Can you work these out from the model? Positions are in its coordinate system, mm. Face numbers are marked on the shaded views. A direction names the side the tool comes from. Coordinates: 2 decimals unless noted, no trailing zeros. Order: outer loops, then holes, each group sorted by start corner. A loop starts at its lowest first (then second) coordinate and runs counter-clockwise, first axis right, second up. Notation, with made-up numbers: (22.25, 16) -> (73.25, 16) arc R13 cw to (73.25, 41) -> close; hole circle Ø1 at (0, 69.25). An arc over 180 degrees is marked (long way). Use a Markdown table: item, result. Add a question column.
1. Suppose I cut it at B-B, the plane z = -12. List the corners of the cut face in (x, y) for me.
2. We'd pull the mould along Z, two halves only. Please class the marked faces 3, 4 and 5: pulls with the +Z half, pulls with the -Z half, needs draft (parallel to the pull), parting line crosses it, or undercut.
3. If I drill on line 1 along Y through (x, z) = (-28.5, -2); line 2 along Y through (x, z) = (35, -16); line 3 along Z through (x, y) = (-12.5, 304), over which ranges is the centre line in solid material (lowest first)? Write a range as from..to.
4. Suppose I cut it at C-C, the plane x = 0. List the corners of the cut face in (y, z) for me.
5. For the marked faces 1 and 2, which set-ups out of +Z, -Z, +X, -X, +Y, -Y let a thin tool reach every point of the face, with its end or its side?
6. For pin 1 Ø2 at (y, z) = (340, 31.5) entering from +X; pin 2 Ø12 at (y, z) = (303.5, -22) entering from +X; pin 3 Ø5.5 at (y, z) = (42.5, 26.5) entering from -X; pin 4 Ø5 at (x, z) = (-13.5, 31.5) entering from -Y, each with a flat end and sliding along its axis, tell me the tip position at first contact or that it passes through.
7. Suppose I cut it at D-D, the plane y = 258. List the corners of the cut face in (x, z) for me.
8. Suppose I cut it at A-A, the plane y = 320.5. List the corners of the cut face in (x, z) for me.
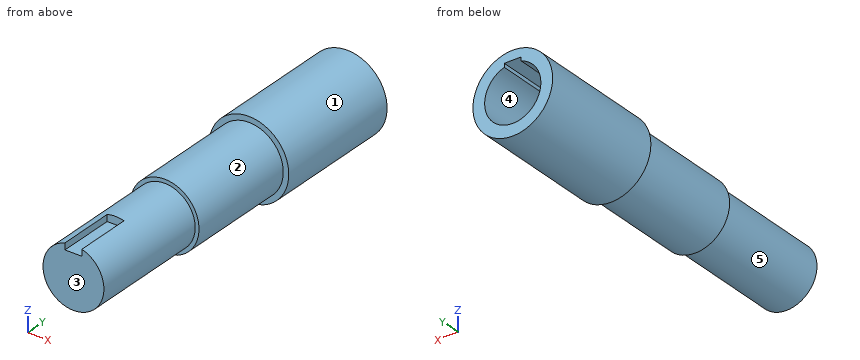
```python
from build123d import *

# Parameters (mm, degrees)
F0_R      = 32.5
F1_DEPTH  = 100
F2_R      = 36.5851523514
F3_DEPTH  = 150
F4_R      = 42.5
F5_DEPTH  = 140
F7_DEPTH  = 110
F9_DEPTH  = 60
F10_R     = 36.5851523514
F10_R_2   = 32.5
F11_DEPTH = 30


with BuildPart() as f1:
    # F0 (on Front) → F1 (new body)
    with BuildSketch(Plane.XZ):
        Circle(F0_R)
    extrude(amount=-F1_DEPTH)

    # F2 (on face) → F3 (join)
    with BuildSketch(Plane(origin=(0, 100, 0), x_dir=(-1, 0, 0), z_dir=(0, 1, 0))):
        Circle(F2_R)
    extrude(amount=F3_DEPTH)

    # F4 (on face) → F5 (join)
    with BuildSketch(Plane(origin=(0, 250, 0), x_dir=(-1, 0, 0), z_dir=(0, 1, 0))):
        Circle(F4_R)
    extrude(amount=F5_DEPTH)

    # F6 (on face) → F7 (cut)
    with BuildSketch(Plane(origin=(0, 390, 0), x_dir=(-1, 0, 0), z_dir=(0, 1, 0))):
        with BuildLine():
            Line((-9, 32.6181760425), (-9, 28.6181760425))
            ThreePointArc((-9, 28.6181760425), (0, -30), (9, 28.6181760425))
            Line((9, 28.6181760425), (9, 32.6181760425))
            Line((9, 32.6181760425), (-9, 32.6181760425))
        make_face()
    extrude(amount=-F7_DEPTH, mode=Mode.SUBTRACT)

    # F8 (on face) → F9 (cut)
    with BuildSketch(Plane.XZ):
        with BuildLine():
            ThreePointArc((9, 31.2289929393), (0, 32.5), (-9, 31.2289929393))
            Line((-9, 31.2289929393), (-9, 24.2289929393))
            Line((-9, 24.2289929393), (9, 24.2289929393))
            Line((9, 24.2289929393), (9, 31.2289929393))
        make_face()
    extrude(amount=-F9_DEPTH, mode=Mode.SUBTRACT)

    # F10 (on face) → F11 (cut)
    with BuildSketch(Plane.XZ.offset(-100)):
        Circle(F10_R)
        Circle(F10_R_2, mode=Mode.SUBTRACT)
    extrude(amount=-F11_DEPTH, mode=Mode.SUBTRACT)


solid = f1.part
```
Worked out:
| question | item | result |
|---|---|---|
| 1 | outline | (-40.77, 250) -> (-34.56, 250) -> (-34.56, 130) -> (-30.2, 130) -> (-30.2, 0) -> (30.2, 0) -> (30.2, 130) -> (34.56, 130) -> (34.56, 250) -> (40.77, 250) -> (40.77, 390) -> (27.5, 390) -> (27.5, 280) -> (-27.5, 280) -> (-27.5, 390) -> (-40.77, 390) -> close |
| 2 | face 3 | needs draft |
| 2 | face 4 | undercut |
| 2 | face 5 | parting line crosses it |
| 3 | line 1 | y = 0..280 |
| 3 | line 2 | y = 250..390 |
| 3 | line 3 | z = -40.62..-27.27, 27.27..40.62 |
| 4 | outline | (0, -32.5) -> (130, -32.5) -> (130, -36.59) -> (250, -36.59) -> (250, -42.5) -> (390, -42.5) -> (390, -30) -> (280, -30) -> (280, 32.62) -> (390, 32.62) -> (390, 42.5) -> (250, 42.5) -> (250, 36.59) -> (130, 36.59) -> (130, 32.5) -> (60, 32.5) -> (60, 24.23) -> (0, 24.23) -> close |
| 5 | face 1 | +Y, -Y |
| 5 | face 2 | -Y |
| 6 | pin 1 | stops at x = 29.6 |
| 6 | pin 2 | stops at x = 39.37 |
| 6 | pin 3 | stops at x = -22.19 |
| 6 | pin 4 | stops at y = 0 |
| 7 | outline | circle Ø85 at (0, 0) |
| 8 | outline | circle Ø85 at (0, 0); hole (-9, 28.62) arc R30 ccw (long way) to (9, 28.62) -> (9, 32.62) -> (-9, 32.62) -> close |
